Geometry: final body of the model. Coordinates: model frame, mm. Give positions to 0.01 mm unless a question says otherwise; leave off trailing zeros. Write each loop counter-clockwise with the first axis right and the second up, starting at its lowest first coordinate (ties: lowest second). Pieces come first, ordered by that corner, then holes. Notation, with made-up numbers: M 24.5,0 L 47.5,0 A18 ccw 47.5,4 Z; hole C 13,-35.5 d9. An arc over 180 degrees is marked long. Answer as a JSON object with one key per item and string values.
from build123d import *

# Parameters (mm, degrees)
ESQUISSE1_R        = 0.875
ESQUISSE1_R_2      = 1.5
ESQUISSE1_R_3      = 3
BOSS_EXTRU_1_DEPTH = 5


with BuildPart() as part:
    # Esquisse1 → Boss.-Extru.1 (new body)
    with BuildSketch(Plane.XY):
        with BuildLine():
            Line((-70, -10), (-0.075038305, -10.499731866))
            ThreePointArc((-0.075038305, -10.499731866), (10.5, 2.989e-05), (-0.075098083, 10.499731438))
            Line((-0.075098083, 10.499731438), (-69.957164253, 9.999908255))
            ThreePointArc((-69.957164253, 9.999908255), (-79.999977064, 0.021417923), (-70, -10))
        make_face()
        with Locations((7.2545, 3.65)):
            Circle(ESQUISSE1_R, mode=Mode.SUBTRACT)
        with Locations((7.2545, 0)):
            Circle(ESQUISSE1_R, mode=Mode.SUBTRACT)
        with Locations(Location((7.2545, -3.65, 0), (0, 0, 180))):
            Circle(ESQUISSE1_R, mode=Mode.SUBTRACT)
        with Locations((3.65, -7.2545)):
            Circle(ESQUISSE1_R, mode=Mode.SUBTRACT)
        with Locations((0, -7.2545)):
            Circle(ESQUISSE1_R, mode=Mode.SUBTRACT)
        with Locations(Location((-3.65, -7.2545, 0), (0, 0, 180))):
            Circle(ESQUISSE1_R, mode=Mode.SUBTRACT)
        with Locations((-7.2545, -3.65)):
            Circle(ESQUISSE1_R, mode=Mode.SUBTRACT)
        with Locations((-7.2545, 0)):
            Circle(ESQUISSE1_R, mode=Mode.SUBTRACT)
        with Locations(Location((-7.2545, 3.65, 0), (0, 0, 180))):
            Circle(ESQUISSE1_R, mode=Mode.SUBTRACT)
        with Locations((-3.65, 7.2545)):
            Circle(ESQUISSE1_R, mode=Mode.SUBTRACT)
        with Locations((0, 7.2545)):
            Circle(ESQUISSE1_R, mode=Mode.SUBTRACT)
        with Locations(Location((3.65, 7.2545, 0), (0, 0, 180))):
            Circle(ESQUISSE1_R, mode=Mode.SUBTRACT)
        with Locations((-70, 0)):
            Circle(ESQUISSE1_R_2, mode=Mode.SUBTRACT)
        with Locations((-40, 0)):
            Circle(ESQUISSE1_R_2, mode=Mode.SUBTRACT)
        Circle(ESQUISSE1_R_3, mode=Mode.SUBTRACT)
    extrude(amount=BOSS_EXTRU_1_DEPTH)


solid = part.part
1) Cut plane A-A on y = 0. Return loops of the section in (x, z).
Geometry check:
{"outline": "M -80,0 L -71.5,0 L -71.5,5 L -80,5 Z; M -68.5,0 L -41.5,0 L -41.5,5 L -68.5,5 Z; M -38.5,0 L -8.13,0 L -8.13,5 L -38.5,5 Z; M -6.38,0 L -3,0 L -3,5 L -6.38,5 Z; M 3,0 L 6.38,0 L 6.38,5 L 3,5 Z; M 8.13,0 L 10.5,0 L 10.5,5 L 8.13,5 Z"}
2) Line query: line 1 (Y direction, x = 0, z = 2.9); line 2 (X direction, y = 6.5, z = 1.7); line 3 (Y direction, x = 3.65, z = 1.85). Output: solid intervals per line, ascending. Write a range as from..to.
Geometry check:
{"line 1": "y = -10.5..-8.13, -6.38..-3, 3..6.38, 8.13..10.5", "line 2": "x = -77.6..-4.09, -3.21..-0.44, 0.44..3.21, 4.09..8.25", "line 3": "y = -9.85..-8.13, -6.38..6.38, 8.13..9.85"}
3) Cut plane C-C on z = 1.7. Give the number of separate pieces and of enclosed holes in the cut face, and give its area (3 significant figures).
Geometry check:
{"separate pieces": "1", "enclosed holes": "15", "area": "1,690 mm2"}
4) Cut plane B-B on x = -40. Return loops of the section in (y, z), and give its area (3 significant figures).
Geometry check:
{"outline": "M -10.21,0 L -1.5,0 L -1.5,5 L -10.21,5 Z; M 1.5,0 L 10.21,0 L 10.21,5 L 1.5,5 Z", "area": "87.1 mm2"}
5) Contact query for flat-ended pins moving along their axis: P1, Ø1.4, axis at x = 3.65, y = -7.25, coming from the -Z side; P2, Ø1.5, axis at x = -68, z = 0.5, coming from the +Y side; P3, Ø1.5, axis at x = -62.5, z = 4, coming from the -Y side; P4, Ø1.5, axis at y = -1, z = 2.5, coming from the +X side. Output: stop coordinate, or through.
Geometry check:
{"P1": "passes through", "P2": "stops at y = 10.02", "P3": "stops at y = -10.06", "P4": "stops at x = 10.5"}
6) Pull-direction query (X, two-part tool) for faces 1 (the flat face through (-35, 0, 0)), 2 (the cylindrical face through (-0.19, 6.4, 2.46)); classes: pulls with the +X half, pulls with the -X half, needs draft (parallel to the pull), parting line crosses it, or undercut.
Geometry check:
{"face 1": "needs draft", "face 2": "undercut"}
